For this review, take the finished solid that the model builds, in its own axes (mm). A direction names the side the tool comes from. Give positions to 0.01 mm unless a question says otherwise; leave off trailing zeros. Loops run counter-clockwise (first coordinate to the right, second up) from the corner with the lowest first, then second, coordinate; pieces in that order, holes last.
```python
from build123d import *

# Parameters (mm, degrees)
SKETCH1_W               = 308
SKETCH1_H               = 95
BOSS_EXTRUDE1_DEPTH     = 270
FILLET1_R               = 30
SKETCH2_OUTSIDE_W       = 394.092
SKETCH2_OUTSIDE_H       = 356.092
CUT_EXTRUDE1_DEPTH      = 421.462840213
FILLET2_R               = 30
CUT_EXTRUDE2_DEPTH      = 413.33511864
CUT_EXTRUDE2_DEPTH_BACK = 413.33511864
SKETCH3_R               = 2.5


with BuildPart() as part:
    # Sketch1 → Boss-Extrude1 (new body)
    with BuildSketch(Plane(origin=(0, 0, 0), x_dir=(1, 0, 0), z_dir=(0, 1, 0))):
        with Locations((-154, 0)):
            Rectangle(SKETCH1_W, SKETCH1_H)
    extrude(amount=BOSS_EXTRUDE1_DEPTH)

    # Fillet1
    fillet1_edges = [part.edges().sort_by_distance(p)[0] for p in [
        (-308, 135, -47.5),
        (0, 135, -47.5),
        (0, 135, 47.5),
        (-308, 135, 47.5),
    ]]
    fillet(fillet1_edges, radius=FILLET1_R)

    # Sketch2 outside → Cut-Extrude1 (cut, through all)
    with BuildSketch(Plane.XY.offset(47.5)):
        with Locations((-154, 135)):
            Rectangle(SKETCH2_OUTSIDE_W, SKETCH2_OUTSIDE_H)
        with BuildLine():
            Line((-228, 0), (-228, 15))
            add(Edge.make_bspline(
                [(-228, 15), (-211.229646979, 15.3677709), (-194.459293959, 15.735541799)],
                knots=[0, 0, 0, 0.14710836, 0.14710836, 0.14710836], degree=2))
            add(Edge.make_bspline(
                [(-194.459293959, 15.735541799), (-97.174631898, -17.834493168), (0, 20)],
                knots=[0, 0, 0, 1, 1, 1], degree=2))
            Line((0, 20), (0, 35))
            Line((0, 35), (-8.156845185, 35))
            Line((-8.156845185, 35), (0, 65.897747125))
            Line((0, 65.897747125), (-135.594672757, 101.694038328))
            Line((-135.594672757, 101.694038328), (-135.594672757, 270))
            Line((-135.594672757, 270), (-310, 270))
            Line((-310, 270), (-292.695445045, 89.818838494))
            Line((-292.695445045, 89.818838494), (-308, 65.708414359))
            Line((-308, 65.708414359), (-308, 0))
            Line((-308, 0), (-228, 0))
        make_face(mode=Mode.SUBTRACT)
    extrude(amount=-CUT_EXTRUDE1_DEPTH, mode=Mode.SUBTRACT)

    # Fillet2
    # the kernel refuses this fillet: 30 mm, written as the material it takes off along each edge
    with BuildSketch(Plane(origin=(-208.110304148, 120.83778937, -47.5), x_dir=(-0.2552500139062178, -0.9668750852105331, 0), z_dir=(0.9668750852105331, -0.2552500139062178, 0))) as fillet2_piece_1_section:
        with BuildLine():
            CenterArc((FILLET2_R, -FILLET2_R), FILLET2_R, 90, 90)
            Line((0, -FILLET2_R), (0, 0))
            Line((0, 0), (FILLET2_R, 0))
        make_face()
    fillet2_piece_1 = extrude(amount=259.212321604, mode=Mode.PRIVATE)
    fillet2_piece_1 = split(fillet2_piece_1, bisect_by=Plane(origin=(-135.594672757, 71.448800887, -40.672385081), z_dir=(1, 0, 0)), keep=Keep.TOP, mode=Mode.PRIVATE)
    add(fillet2_piece_1, mode=Mode.SUBTRACT)
    with BuildSketch(Plane(origin=(42.515631391, 54.673840676, 47.5), x_dir=(0, 0, -1), z_dir=(-0.9668750852105331, 0.2552500139062178, 0))) as fillet2_piece_2_section:
        with BuildLine():
            CenterArc((FILLET2_R, FILLET2_R), FILLET2_R, 180, 90)
            Line((0, FILLET2_R), (0, 0))
            Line((0, 0), (FILLET2_R, 0))
        make_face()
    fillet2_piece_2 = extrude(amount=259.212321604, mode=Mode.PRIVATE)
    fillet2_piece_2 = split(fillet2_piece_2, bisect_by=Plane(origin=(-135.594672757, 71.448800887, 40.672385081), z_dir=(1, 0, 0)), keep=Keep.TOP, mode=Mode.PRIVATE)
    add(fillet2_piece_2, mode=Mode.SUBTRACT)
    with BuildSketch(Plane(origin=(-135.594672757, 345, -47.5), x_dir=(-1, 0, 0), z_dir=(0, -1, 0))) as fillet2_piece_3_section:
        with BuildLine():
            CenterArc((FILLET2_R, -FILLET2_R), FILLET2_R, 90, 90)
            Line((0, -FILLET2_R), (0, 0))
            Line((0, 0), (FILLET2_R, 0))
        make_face()
    fillet2_piece_3 = extrude(amount=318.305961672, mode=Mode.PRIVATE)
    fillet2_piece_3 = split(fillet2_piece_3, bisect_by=Plane(origin=(-172.144372256, 111.342969661, -40.68113524), z_dir=(0.2552500139062178, 0.9668750852105331, 0)), keep=Keep.TOP, mode=Mode.PRIVATE)
    add(fillet2_piece_3, mode=Mode.SUBTRACT)
    with BuildSketch(Plane(origin=(-135.594672757, 26.694038328, 47.5), x_dir=(0, 0, -1), z_dir=(0, 1, 0))) as fillet2_piece_4_section:
        with BuildLine():
            CenterArc((FILLET2_R, FILLET2_R), FILLET2_R, 180, 90)
            Line((0, FILLET2_R), (0, 0))
            Line((0, 0), (FILLET2_R, 0))
        make_face()
    fillet2_piece_4 = extrude(amount=318.305961672, mode=Mode.PRIVATE)
    fillet2_piece_4 = split(fillet2_piece_4, bisect_by=Plane(origin=(-172.144372256, 111.342969661, 40.68113524), z_dir=(0.2552500139062178, 0.9668750852105331, 0)), keep=Keep.TOP, mode=Mode.PRIVATE)
    add(fillet2_piece_4, mode=Mode.SUBTRACT)
    with BuildSketch(Plane(origin=(-208.110304148, 120.83778937, -47.5), x_dir=(-0.2552500139062178, -0.9668750852105331, 0), z_dir=(0.9668750852105331, -0.2552500139062178, 0))) as fillet2_piece_5a_section:
        with BuildLine():
            CenterArc((FILLET2_R, -FILLET2_R), FILLET2_R, 90, 90)
            Line((0, -FILLET2_R), (0, 0))
            Line((0, 0), (FILLET2_R, 0))
        make_face()
    fillet2_piece_5a = extrude(amount=259.212321604, mode=Mode.PRIVATE)
    fillet2_piece_5a = split(fillet2_piece_5a, bisect_by=Plane(origin=(-135.594672757, 104.326327601, -40.79309683), z_dir=(-1, 0, 0)), keep=Keep.TOP, mode=Mode.PRIVATE)
    with BuildSketch(Plane(origin=(-135.594672757, 345, -47.5), x_dir=(-1, 0, 0), z_dir=(0, -1, 0))) as fillet2_piece_5b_section:
        with BuildLine():
            CenterArc((FILLET2_R, -FILLET2_R), FILLET2_R, 90, 90)
            Line((0, -FILLET2_R), (0, 0))
            Line((0, 0), (FILLET2_R, 0))
        make_face()
    fillet2_piece_5b = extrude(amount=318.305961672, mode=Mode.PRIVATE)
    fillet2_piece_5b = split(fillet2_piece_5b, bisect_by=Plane(origin=(-133.049577842, 101.022146454, -40.79309683), z_dir=(-0.2552500139062178, -0.9668750852105331, 0)), keep=Keep.TOP, mode=Mode.PRIVATE)
    fillet2_piece_5 = fillet2_piece_5a & fillet2_piece_5b
    add(fillet2_piece_5, mode=Mode.SUBTRACT)
    with BuildSketch(Plane(origin=(42.515631391, 54.673840676, 47.5), x_dir=(0, 0, -1), z_dir=(-0.9668750852105331, 0.2552500139062178, 0))) as fillet2_piece_6a_section:
        with BuildLine():
            CenterArc((FILLET2_R, FILLET2_R), FILLET2_R, 180, 90)
            Line((0, FILLET2_R), (0, 0))
            Line((0, 0), (FILLET2_R, 0))
        make_face()
    fillet2_piece_6a = extrude(amount=259.212321604, mode=Mode.PRIVATE)
    fillet2_piece_6a = split(fillet2_piece_6a, bisect_by=Plane(origin=(-135.594672757, 104.326327601, 40.79309683), z_dir=(-1, 0, 0)), keep=Keep.TOP, mode=Mode.PRIVATE)
    with BuildSketch(Plane(origin=(-135.594672757, 26.694038328, 47.5), x_dir=(0, 0, -1), z_dir=(0, 1, 0))) as fillet2_piece_6b_section:
        with BuildLine():
            CenterArc((FILLET2_R, FILLET2_R), FILLET2_R, 180, 90)
            Line((0, FILLET2_R), (0, 0))
            Line((0, 0), (FILLET2_R, 0))
        make_face()
    fillet2_piece_6b = extrude(amount=318.305961672, mode=Mode.PRIVATE)
    fillet2_piece_6b = split(fillet2_piece_6b, bisect_by=Plane(origin=(-133.049577842, 101.022146454, 40.79309683), z_dir=(-0.2552500139062178, -0.9668750852105331, 0)), keep=Keep.TOP, mode=Mode.PRIVATE)
    fillet2_piece_6 = fillet2_piece_6a & fillet2_piece_6b
    add(fillet2_piece_6, mode=Mode.SUBTRACT)

    # Sketch3 → Cut-Extrude2 (cut, two sides: drawn at the far end of the back side and taken through both)
    with BuildSketch(Plane.XY.offset(-CUT_EXTRUDE2_DEPTH_BACK)):
        with Locations((-15, 25.4)):
            Circle(SKETCH3_R)
    extrude(amount=CUT_EXTRUDE2_DEPTH + CUT_EXTRUDE2_DEPTH_BACK, mode=Mode.SUBTRACT)


solid = part.part
```
Q1. Machinability: for faces 5 (the flat face through (-300.24, 77.93, 0.61)), 6 (the flat face through (-135.595, 185, 0)), 7 (the flat face through (-4, 35, 1)), which of the approach directions +Z, -Z, +X, -X, +Y, -Y give a long, thin tool a straight path to every point of the face, cutting with its end or side? Answer none if there is none.
Answers:
face 5: +Z, -Z, -X
face 6: +Z, -Z, +X, +Y
face 7: +Z, -Z, +X
Q2. Consider section A-A on y = 175.5. Give the boundary of the cut face in (x, z).
Answers:
outline: (-300.92, -36.85) arc R30 ccw to (-278, -47.5) - (-165.59, -47.5) arc R30 ccw to (-135.59, -17.5) - (-135.59, 17.5) arc R30 ccw to (-165.59, 47.5) - (-278, 47.5) arc R30 ccw to (-300.92, 36.85) - close
Q3. For pin 1 Ø8 at (y, z) = (95.5, -4.5) entering from -X; pin 2 Ø4 at (x, z) = (-4, -6) entering from +Y; pin 3 Ø1.5 at (y, z) = (214.5, 11) entering from +X; pin 4 Ø4 at (x, y) = (-15, 25.4) entering from +Z, all flat-tipped, find the tip position at first contact; note any pin that passes through.
Answers:
pin 1: stops at x = -293.63
pin 2: stops at y = 67.48
pin 3: stops at x = -135.59
pin 4: passes through
Q4. For probe 1 along X at (y, z) = (25, 12); probe 2 along Y at (x, z) = (-15, 6); probe 3 along Z at (x, y) = (-280, 222), list the stretches that pass through material, from the lowest coordinate up.
Answers:
probe 1: x = -308 to -17.47, -12.53 to 0
probe 2: y = 14.59 to 22.9, 27.9 to 69.86
probe 3: z = -47.43 to 47.43
Q5. Mouldability with a two-part tool opening along X and no side actions: class faces 1 (the cylindrical face through (-295.48, 136.89, -41.88)), 2 (the cylindrical face through (-144.62, 175.63, -38.95)), 3 (the flat face through (-183, 103, -47.5)), 4 (the flat face through (-228, 7, 1)) as +X half, -X half, draft (parallel to the pull), parting line (faces both ways), or undercut.
Answers:
face 1: -X half
face 2: +X half
face 3: draft
face 4: undercut
